```python
from build123d import *

# Parameters (mm, degrees)
SKETCH_W      = 50
SKETCH_H      = 300
PAD_DEPTH     = 3
SKETCH001_R   = 10
SKETCH001_W   = 3
SKETCH001_H   = 20
SKETCH001_W_2 = 8
SKETCH001_H_2 = 3
POCKET_DEPTH  = 3.001


with BuildPart() as part:
    # Sketch → Pad (new body)
    with BuildSketch(Plane.XY):
        with Locations((25, 150)):
            Rectangle(SKETCH_W, SKETCH_H)
    extrude(amount=PAD_DEPTH)

    # Sketch001 (on Face6 of Pad) → Pocket (cut, through all)
    with BuildSketch(Plane.XY.offset(3)):
        with Locations((31, 52)):
            Circle(SKETCH001_R)
        with Locations((31, 132)):
            Circle(SKETCH001_R)
        with Locations((31, 212)):
            Circle(SKETCH001_R)
        with Locations((1.5, 30)):
            Rectangle(SKETCH001_W, SKETCH001_H)
        with Locations((1.5, 70)):
            Rectangle(SKETCH001_W, SKETCH001_H)
        with Locations((1.5, 110)):
            Rectangle(SKETCH001_W, SKETCH001_H)
        with Locations((1.5, 150)):
            Rectangle(SKETCH001_W, SKETCH001_H)
        with Locations((1.5, 190)):
            Rectangle(SKETCH001_W, SKETCH001_H)
        with Locations((1.5, 230)):
            Rectangle(SKETCH001_W, SKETCH001_H)
        with Locations((1.5, 270)):
            Rectangle(SKETCH001_W, SKETCH001_H)
        with Locations((14.5, 30)):
            Rectangle(SKETCH001_W, SKETCH001_H)
        with Locations((14.5, 70)):
            Rectangle(SKETCH001_W, SKETCH001_H)
        with Locations((14.5, 110)):
            Rectangle(SKETCH001_W, SKETCH001_H)
        with Locations((14.5, 150)):
            Rectangle(SKETCH001_W, SKETCH001_H)
        with Locations((14.5, 190)):
            Rectangle(SKETCH001_W, SKETCH001_H)
        with Locations((14.5, 230)):
            Rectangle(SKETCH001_W, SKETCH001_H)
        with Locations((14.5, 270)):
            Rectangle(SKETCH001_W, SKETCH001_H)
        with Locations((48.5, 30)):
            Rectangle(SKETCH001_W, SKETCH001_H)
        with Locations((48.5, 70)):
            Rectangle(SKETCH001_W, SKETCH001_H)
        with Locations((48.5, 110)):
            Rectangle(SKETCH001_W, SKETCH001_H)
        with Locations((48.5, 150)):
            Rectangle(SKETCH001_W, SKETCH001_H)
        with Locations((48.5, 190)):
            Rectangle(SKETCH001_W, SKETCH001_H)
        with Locations((48.5, 230)):
            Rectangle(SKETCH001_W, SKETCH001_H)
        with Locations((48.5, 270)):
            Rectangle(SKETCH001_W, SKETCH001_H)
        with Locations((1, 1.5)):
            Rectangle(SKETCH001_W_2, SKETCH001_H_2)
        with Locations((17, 1.5)):
            Rectangle(SKETCH001_W_2, SKETCH001_H_2)
        with Locations((33, 1.5)):
            Rectangle(SKETCH001_W_2, SKETCH001_H_2)
        with Locations((49, 1.5)):
            Rectangle(SKETCH001_W_2, SKETCH001_H_2)
        with Locations((1, 298.5)):
            Rectangle(SKETCH001_W_2, SKETCH001_H_2)
        with Locations((17, 298.5)):
            Rectangle(SKETCH001_W_2, SKETCH001_H_2)
        with Locations((33, 298.5)):
            Rectangle(SKETCH001_W_2, SKETCH001_H_2)
        with Locations((49, 298.5)):
            Rectangle(SKETCH001_W_2, SKETCH001_H_2)
    extrude(amount=-POCKET_DEPTH, mode=Mode.SUBTRACT)


solid = part.part
```
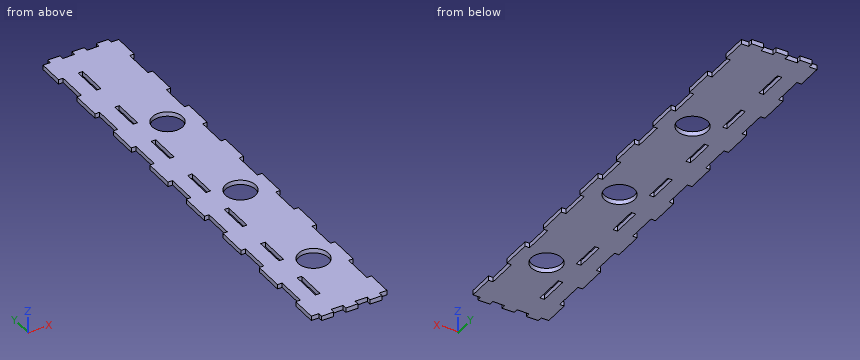
Work out the finished part from the listing and answer in its coordinate system (mm). Round coordinates to 2 decimals unless told otherwise and drop trailing zeros. Order: outer loops, then holes, each group sorted by start corner. A loop starts at its lowest first (then second) coordinate and runs counter-clockwise, first axis right, second up.
Q1. Given pin 1 Ø1.5 at (y, z) = (269, 2) entering from +X; pin 2 Ø0.9 at (x, z) = (15, 2) entering from -Y; pin 3 Ø0.9 at (y, z) = (106, 2) entering from -X, each flat-ended and moving along its own axis, determine where each tip first touches the part or whether it passes through.
Solution:
pin 1: stops at x = 47
pin 2: stops at y = 3
pin 3: stops at x = 3
Q2. A cutting plane is placed at A-A, the plane y = 212. Determine the outline of the cut face in (x, z), then the cut area to 3 significant figures.
Solution:
outline: (0, 0) - (21, 0) - (21, 3) - (0, 3) - close; (41, 0) - (50, 0) - (50, 3) - (41, 3) - close
area: 90.0 mm2
Q3. A cutting plane is placed at B-B, the plane x = 23.5. Determine the outline of the cut face in (y, z), then the cut area to 3 significant figures.
Solution:
outline: (0, 0) - (45.39, 0) - (45.39, 3) - (0, 3) - close; (58.61, 0) - (125.39, 0) - (125.39, 3) - (58.61, 3) - close; (138.61, 0) - (205.39, 0) - (205.39, 3) - (138.61, 3) - close; (218.61, 0) - (300, 0) - (300, 3) - (218.61, 3) - close
area: 781 mm2
Q4. A cutting plane is placed at D-D, the plane z = 1.95. Count the separate pieces of the cut face and the enclosed holes in it, then the cut area to 3 significant figures.
Solution:
separate pieces: 1
enclosed holes: 10
area: 12,600 mm2
Q5. Find the intervals of material crossed by line 1 along Y through (x, z) = (31, 1.9); line 2 along X through (y, z) = (227, 2.75); line 3 along Y through (x, z) = (38, 0.35), in increasing order.
Solution:
line 1: y = 3 to 42, 62 to 122, 142 to 202, 222 to 297
line 2: x = 3 to 13, 16 to 47
line 3: y = 0 to 44.86, 59.14 to 124.86, 139.14 to 204.86, 219.14 to 300
Q6. A cutting plane is placed at C-C, the plane y = 35.5. Determine the outline of the cut face in (x, z), then the cut area to 3 significant figures.
Solution:
outline: (3, 0) - (13, 0) - (13, 3) - (3, 3) - close; (16, 0) - (47, 0) - (47, 3) - (16, 3) - close
area: 123 mm2
